Read the model definition and answer for the solid it produces. Units are mm, in the model's axes. Give positions to 0.01 mm unless a question says otherwise; leave off trailing zeros. Order: outer loops, then holes, each group sorted by start corner. A loop starts at its lowest first (then second) coordinate and runs counter-clockwise, first axis right, second up. Notation, with made-up numbers: M 11,2 L 55,2 A35 ccw 55,40 Z; hole C 58.5,47 d6. An arc over 180 degrees is marked long. One line per item, written item: value.
from build123d import *

# Parameters (mm, degrees)
SKETCH_1_R      = 3
SKETCH_1_R_2    = 5
EXTRUDE_1_DEPTH = 5


with BuildPart() as part:
    # 草图1 → 凸台-拉伸1 (new, symmetric)
    with BuildSketch(Plane(origin=(0, 0, 0), x_dir=(1, 0, 0), z_dir=(0, 1, 0))):
        with BuildLine():
            Line((-54.060747664, 5.97373937), (-1.028037383, 10.951855511))
            ThreePointArc((-1.028037383, 10.951855511), (-0.23963625, 10.997389439), (0.55, 10.986241395))
            Line((0.55, 10.986241395), (100.3, 5.992495307))
            ThreePointArc((100.3, 5.992495307), (106, 0), (100.3, -5.992495307))
            Line((100.3, -5.992495307), (0.55, -10.986241395))
            ThreePointArc((0.55, -10.986241395), (-0.23963625, -10.997389439), (-1.028037383, -10.951855511))
            Line((-1.028037383, -10.951855511), (-54.060747664, -5.97373937))
            ThreePointArc((-54.060747664, -5.97373937), (-59.5, 0), (-54.060747664, 5.97373937))
        make_face()
        with Locations(Location((-53.5, 0, 0), (0, 0, 270))):
            Circle(SKETCH_1_R, mode=Mode.SUBTRACT)
        with Locations(Location((100, 0, 0), (0, 0, 270))):
            Circle(SKETCH_1_R, mode=Mode.SUBTRACT)
        with Locations(Location((0, 0, 0), (0, 0, 270))):
            Circle(SKETCH_1_R_2, mode=Mode.SUBTRACT)
    extrude(amount=EXTRUDE_1_DEPTH, both=True)


solid = part.part
1) Find section B-B, the plane y = 3.25. Write down the section's boundary in (x, z), plus the area to 3 significant figures.
Reported:
outline: M -54.06,-5.97 L -1.03,-10.95 A11 ccw 0.55,-10.99 L 100.3,-5.99 A6 ccw 100.3,5.99 L 0.55,10.99 A11 ccw -1.03,10.95 L -54.06,5.97 A6 ccw Z; hole C -53.5,0 d6; hole C 0,0 d10; hole C 100,0 d6
area: 2,590 mm^2
2) Find section C-C, the plane x = 24. Write down the section's boundary in (y, z).
Reported:
outline: M -5,-9.81 L 5,-9.81 L 5,9.81 L -5,9.81 Z
3) Find section D-D, the plane x = 54.5. Write down the section's boundary in (y, z).
Reported:
outline: M -5,-8.29 L 5,-8.29 L 5,8.29 L -5,8.29 Z
4) Find section A-A, the plane z = 0. Write down the section's boundary in (x, y), plus the area to 4 significant figures.
Reported:
outline: M -59.5,-5 L -56.5,-5 L -56.5,5 L -59.5,5 Z; M -50.5,-5 L -5,-5 L -5,5 L -50.5,5 Z; M 5,-5 L 97,-5 L 97,5 L 5,5 Z; M 103,-5 L 106,-5 L 106,5 L 103,5 Z
area: 1,435 mm^2
5) Determine the mould class of faces 1 (the face through (97.07, -0.07, -0.65)), 2 (the face through (-27.173, 0.07, 8.498)), 3 (the face through (106, 0, 0)), 4 (the face through (-4.88, -0.07, -1.08)) for opening direction Z: +Z half, -Z half, draft (parallel to the pull), parting line (faces both ways), or undercut.
Reported:
face 1: undercut
face 2: +Z half
face 3: parting line
face 4: undercut
6) Each of these flat-tipped pins is pushed along its axis until it touches: pin 1 Ø1.5 at (y, z) = (2.5, 2) entering from +X; pin 2 Ø4 at (y, z) = (-3, 5.5) entering from -X; pin 3 Ø3 at (x, y) = (55.5, 1.5) entering from -Z. Where does it stop, or does it pass through?
Reported:
pin 1: stops at x = 105.87
pin 2: stops at x = -58.37
pin 3: stops at z = -8.31
7) Consider probe 1 along X at (y, z) = (0.25, 0); probe 2 along X at (y, z) = (-3.25, 2); probe 3 along X at (y, z) = (0.5, -4). Determine where each line is inside the solid, lowest interval first.
Reported:
probe 1: x = -59.5 to -56.5, -50.5 to -5, 5 to 97, 103 to 106
probe 2: x = -59.16 to -55.74, -51.26 to -4.58, 4.58 to 97.76, 102.24 to 105.66
probe 3: x = -57.97 to -3, 3 to 104.47
